The model under review builds one solid part; all positions refer to its coordinate system, in mm. Face numbers are marked on the shaded views. A direction names the side the tool comes from. Coordinates: 2 decimals unless noted, no trailing zeros. Loops run counter-clockwise (first coordinate to the right, second up) from the corner with the lowest first, then second, coordinate; pieces in that order, holes last. Notation, with made-up numbers: (75.5, 15) - (124.5, 15) arc R30 ccw to (124.5, 47) - close; hole circle Ø8 at (64.25, 59.25). An arc over 180 degrees is marked (long way). Answer in a Markdown table with one row per item. Add a question column.
(1) For line 1 along X through (y, z) = (3, -0.5); line 2 along Z through (x, y) = (32.5, 1.75); line 3 along Z through (x, y) = (8.5, 3), list the stretches that pass through material, from the lowest coordinate up.
(2) For P1, Ø8, axis at y = 2, z = -14, coming from the -X side; P2, Ø6, axis at x = 38.735, z = 12.7, coming from the +Y side (3 decimals); P3, Ø1, axis at y = 10, z = -15, coming from the +X side, all flat-tipped, find the tip position at first contact; note any pin that passes through.
(3) Machinability: for the marked faces 1 and 2, which of the approach directions +Z, -Z, +X, -X, +Y, -Y give a long, thin tool a straight path to every point of the face, cutting with its end or side? Answer none if there is none.
(4) We need section B-B on z = 12.7. Give the number of separate pieces and of enclosed holes in the cut face, plus the area to 3 significant figures.
(5) We need section A-A on x = -35.56. Write out the cut boundary in (y, z) (3 decimals).
Autodesk Inventor part; units mm, degrees
ref_plane "YZ Plane" through (0, 0, 0) normal (1, 0, 0) x (0, 1, 0)
ref_plane "XZ Plane" through (0, 0, 0) normal (0, 1, 0) x (-1, 0, 0)
ref_plane "XY Plane" through (0, 0, 0) normal (0, 0, 1) x (1, 0, 0)
sketch "Sketch1" plane through (0, 0, 0) normal (0, 1, 0) x (-1, 0, 0)
  line L0 (-50.8, -19.05) -> (50.8, -19.05)
  line L1 (50.8, -19.05) -> (50.8, 19.05)
  line L2 (50.8, 19.05) -> (-50.8, 19.05)
  line L3 (-50.8, 19.05) -> (-50.8, -19.05)
  line L4 (-50.8, -19.05) -> (50.8, 19.05) construction
  line L5 (50.8, -19.05) -> (-50.8, 19.05) construction
  point P0 (0, 0)
  dimension "d0" = 38.1
  dimension "d1" = 101.6
extrude "Plate1" add sketch "Sketch1" along normal blind 3.175
sketch "Sketch2" plane through (-48.5549, 2.2451, 19.05) normal (-0.7071068, -0.7071068, 0) x (0.7071068, -0.7071068, 0)
  line L0 (0, -38.1) -> (0, 0)
  line L1 (0, 0) -> (-19.05, 0)
  line L2 (-19.05, 0) -> (-19.05, -38.1)
  line L3 (-19.05, -38.1) -> (0, -38.1)
edge flange "Flange1" height 19.05 angle 45 thickness 3.175 bend radius 3.175 thickness toward (-0.7071068, -0.7071068, 0) relief tear relief width 3.175 relief depth 1.5875 edges at (-50.8, 3.175, 0) wall of the first edge with corners at (-48.5549, 2.2451, -19.05) (-48.5549, 2.2451, 19.05) (-62.0253, 15.7154, 19.05) (-62.0253, 15.7154, -19.05)
bend "Bend1"
corner "Corner1"
sketch "Sketch3" plane through (-62.0253, 15.7154, -19.05) normal (0.7071068, 0.7071068, 0) x (-0.7071068, 0.7071068, 0)
  circle A0 centre (-7.62, 19.05) radius 4.1275
  circle A1 centre (-7.62, 26.9875) radius 1.2446
  circle A2 centre (-7.62, 11.1125) radius 1.2446
  line L0 (-132.4339, 19.05) -> (42.7893, 19.05)
  line L1 (0, 0) -> (0, 38.1)
  point P0 (-54.971, 19.05)
  dimension "d13" = 8.255
  dimension "d14" = 2.4892
  dimension "d15" = 7.9375
  dimension "d16" = 7.9375
  dimension "d17" = 7.62
extrude "Cut1" cut sketch "Sketch3" against normal blind 3.175
sketch "Sketch4" plane through (0, 3.175, 0) normal (0, 1, 0) x (1, 0, 0)
  line L0 (32.385, -12.7) -> (6.985, -12.7)
  line L1 (6.985, -12.7) -> (6.985, 12.7)
  line L2 (6.985, 12.7) -> (32.385, 12.7)
  line L3 (32.385, 12.7) -> (32.385, -12.7)
  line L4 (32.385, -12.7) -> (6.985, 12.7) construction
  line L5 (6.985, -12.7) -> (32.385, 12.7) construction
  line L6 (50.8, 19.05) -> (50.8, -19.05)
  point P0 (0, 0)
  point P1 (19.685, 0)
  point P2 (32.385, -12.7)
  point P3 (38.735, -12.7)
  point P4 (26.035, -12.7)
  point P5 (13.335, -12.7)
  point P6 (0.635, -12.7)
  point P7 (13.335, 12.7)
  point P8 (0.635, 12.7)
  point P9 (26.035, 12.7)
  point P10 (38.735, 12.7)
  point P11 (-35.56, 0)
  point P12 (19.685, 0)
  point P13 (19.685, 0)
  dimension "d20" = 25.4
  dimension "d21" = 25.4
  dimension "d32" = 19.685
  dimension "d33" = 6.35
  dimension "d34" = 6.35
  dimension "d35" = 6.35
  dimension "d36" = 6.35
  dimension "d37" = 35.56
hole "Hole1" at (6.985, 3.175, -12.7) at (32.385, 3.175, -12.7) at (32.385, 3.175, 12.7) at (6.985, 3.175, 12.7) at (38.735, 3.175, 12.7) at (26.035, 3.175, 12.7) at (38.735, 3.175, -12.7) at (13.335, 3.175, -12.7) at (26.035, 3.175, -12.7) at (0.635, 3.175, -12.7) at (0.635, 3.175, 12.7) at (13.335, 3.175, 12.7) direction (0, -1, 0) diameter 4.7625 depth 3.175 tip angle 118
fillet "Corner Round1" radius 3.175 4 edges at (-63.1479, 14.5929, -19.05) (-63.1479, 14.5929, 19.05) (50.8, 1.5875, -19.05) (50.8, 1.5875, 19.05)
sketch "Sketch5" plane through (0, 0, 0) normal (0, 0, 1) x (1, 0, 0)
  line L0 (-104.5658, 0) -> (17.4276, 0)
  line L1 (17.4757, 84.4402) -> (-106.4259, -39.4614)
  line L2 (-52.6599, 1.8599) -> (-62.0253, 11.2253)
  line L3 (-58.8822, 8.0822) -> (-90.3131, -23.3487)
  point P0 (0, 0)
  dimension "d31" = 44.45
hole "Hole2" at (-35.56, 3.175, 0) at (19.685, 3.175, 0) direction (0, -1, 0) diameter 2.4638 end through all
equation "\"d18\" = Thickness"
equation "\"d28\" = Thickness"
equation "\"d3\" = BendReliefWidth"
equation "\"d4\" = BendReliefDepth"
equation "\"d5\" = MinimumRemnant"
equation "\"d6\" = BendRadius"
equation "\"d9\" = BendRadius"
equation "\"d10\" = CornerReliefSize"
equation "\"d11\" = GapSize"
equation "\"d12\" = JacobiRadiusSize"
equation "\"BendRadius\" = Thickness"
equation "\"BendReliefWidth\" = Thickness"
equation "\"BendReliefDepth\" = 0.5 * Thickness"
equation "\"CornerReliefSize\" = 4 * Thickness"
equation "\"MinimumRemnant\" = 2 * Thickness"
equation "\"TransitionRadius\" = BendRadius"
equation "\"JacobiRadiusSize\" = BendRadius"
equation "\"GapSize\" = Thickness"
equation "\"d2\" = BendRadius"
properties part number "J005232" material "ALUMINUM, 5052-H32"
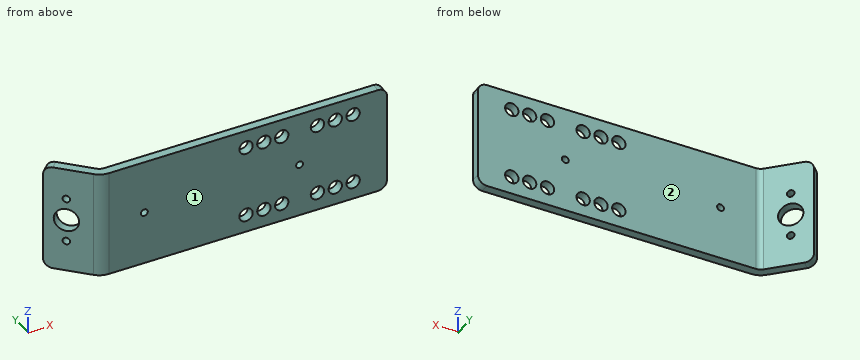
Outcome:
| question | item | result |
|---|---|---|
| 1 | line 1 | -53.8 to -36.69, -34.43 to 18.56, 20.81 to 50.8 |
| 1 | line 2 | -19.05 to -15.08, -10.32 to 10.32, 15.08 to 19.05 |
| 1 | line 3 | -19.05 to -14.54, -10.86 to 10.86, 14.54 to 19.05 |
| 2 | P1 | x = -56.8 |
| 2 | P2 | y = 3.175 |
| 2 | P3 | x = -55.81 |
| 3 | face 1 | +Z, -Z, +X, -X, -Y |
| 3 | face 2 | +Z, -Z, +X, +Y |
| 4 | separate pieces | 7 |
| 4 | enclosed holes | 0 |
| 4 | area | 288 mm² |
| 5 | outline | (0, -19.05) - (3.175, -19.05) - (3.175, -1.232) - (0, -1.232) - close; (0, 1.232) - (3.175, 1.232) - (3.175, 19.05) - (0, 19.05) - close |
